Model file for the job. Use its own axes, mm. A direction names the side the tool comes from. Round coordinates to 2 decimals unless told otherwise and drop trailing zeros. Order: outer loops, then holes, each group sorted by start corner. A loop starts at its lowest first (then second) coordinate and runs counter-clockwise, first axis right, second up. Notation, with made-up numbers: M -1,58 L 54,58 A10 ccw 54,62 Z; hole C 20.25,53.25 d7. An arc over 180 degrees is marked long. Return JSON: item names as keys, results as strings. Group by question number.
Item 1: Slice it at C-C on z = 1.1. Write the cut outline in (x, y), then the cut area to 3 significant figures.
Item 2: Pull direction Y, two halves, no side cores. Call faces 1 (the face through (-9.5, 2.5, 1)), 2 (the face through (0, 22.5, 1)), 3 (the face through (5, 0.5, 1)), 4 (the face through (0, 0, 0)): pulls with the +Y half, pulls with the -Y half, needs draft (parallel to the pull), parting line crosses it, or undercut.
Item 3: Probe line 1 along Y through (x, z) = (-5, 0.95); line 2 along X through (y, z) = (2.5, 1.9); line 3 along X through (y, z) = (4, 1.3). List the from-to ranges inside material, lowest first.
Item 4: Slice it at B-B on x = 16. Write the cut outline in (y, z).
Item 5: Which spindle directions (+Z, -Z, +X, -X, +Y, -Y) get a long thin tool onto all of the face, cutting with end or side? Do faces 5 (the face through (32.5, 0, 1)), 6 (the face through (19.5, 2.5, 1)). Say none if no direction does.
Item 6: Slice it at A-A on y = 2.5. Write the cut outline in (x, z), then the cut area to 3 significant figures.
from build123d import *

# Parameters (mm, degrees)
SKETCH1_W           = 65
SKETCH1_H           = 45
BOSS_EXTRUDE1_DEPTH = 2
CUT_EXTRUDE2_DEPTH  = 2


with BuildPart() as part:
    # Sketch1 → Boss-Extrude1 (new body)
    with BuildSketch(Plane.XY):
        Rectangle(SKETCH1_W, SKETCH1_H)
    extrude(amount=BOSS_EXTRUDE1_DEPTH)

    # Sketch2 → Cut-Extrude2 (cut)
    with BuildSketch(Plane.XY):
        with BuildLine():
            Line((-7.5, 4.5), (17.5, 4.5))
            ThreePointArc((17.5, 4.5), (19.5, 2.5), (17.5, 0.5))
            Line((17.5, 0.5), (-7.5, 0.5))
            ThreePointArc((-7.5, 0.5), (-9.5, 2.5), (-7.5, 4.5))
        make_face()
    extrude(amount=CUT_EXTRUDE2_DEPTH, mode=Mode.SUBTRACT)


solid = part.part
Output values:
{
 "1": {"outline": "M -32.5,-22.5 L 32.5,-22.5 L 32.5,22.5 L -32.5,22.5 Z; hole M -7.5,0.5 L 17.5,0.5 A2 ccw 17.5,4.5 L -7.5,4.5 A2 ccw Z", "area": "2,810 mm²"},
 "2": {"face 1": "undercut", "face 2": "pulls with the +Y half", "face 3": "undercut", "face 4": "needs draft"},
 "3": {"line 1": "-22.5 to 0.5, 4.5 to 22.5", "line 2": "-32.5 to -9.5, 19.5 to 32.5", "line 3": "-32.5 to -8.82, 18.82 to 32.5"},
 "4": {"outline": "M -22.5,0 L 0.5,0 L 0.5,2 L -22.5,2 Z; M 4.5,0 L 22.5,0 L 22.5,2 L 4.5,2 Z"},
 "5": {"face 5": "+Z, -Z, +X, +Y, -Y", "face 6": "+Z, -Z"},
 "6": {"outline": "M -32.5,0 L -9.5,0 L -9.5,2 L -32.5,2 Z; M 19.5,0 L 32.5,0 L 32.5,2 L 19.5,2 Z", "area": "72.0 mm²"}
}
